The drawing under review shows one solid part. Ordinate dimensions are in mm from its lowest x, y, z. Coordinates: 2 decimals unless noted, no trailing zeros. Loops run counter-clockwise (first coordinate to the right, second up) from the corner with the lowest first, then second, coordinate; pieces in that order, holes last. Notation, with made-up numbers: (53, 15) -> (106, 15) arc R18 ccw to (106, 40) -> close; hole circle Ø4 at (22.5, 17). An arc over 180 degrees is marked (long way). Use a Markdown table: item, result.
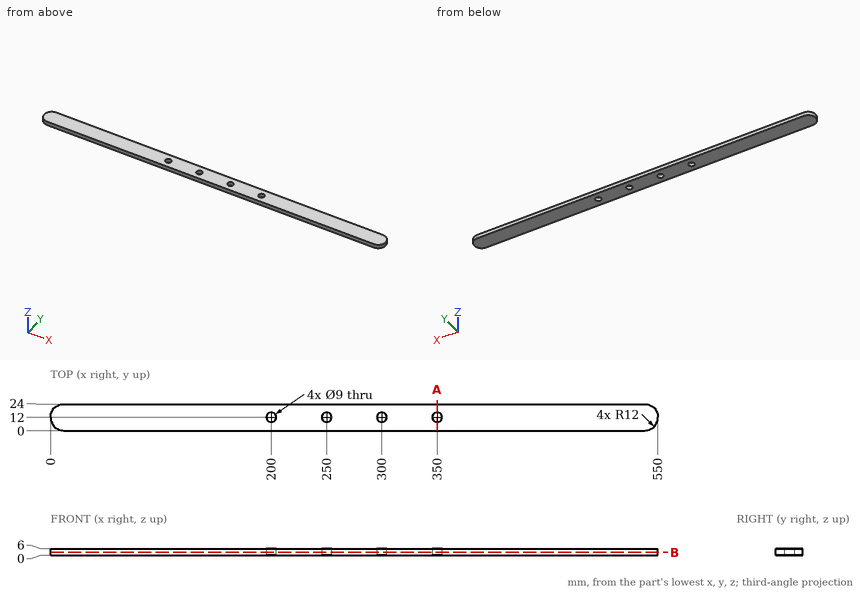
(1) Take a section at B-B on z = 2.45. State how many separate pieces and enclosed holes the cut face has, plus the area to 3 significant figures.
Found:
| item | result |
|---|---|
| separate pieces | 1 |
| enclosed holes | 4 |
| area | 12,800 mm^2 |
(2) For pin 1 Ø1.5 at (y, z) = (6.5, 3) entering from +X; pin 2 Ø1.5 at (y, z) = (16.5, 2.5) entering from -X, all flat-tipped, find the tip position at first contact; note any pin that passes through.
Found:
| item | result |
|---|---|
| pin 1 | stops at x = 549.02 |
| pin 2 | stops at x = 0.6 |
(3) Take a section at A-A on x = 350. Write out the cut boundary in (y, z), plus the area to 3 significant figures.
Found:
| item | result |
|---|---|
| outline | (0, 0) -> (7.5, 0) -> (7.5, 6) -> (0, 6) -> close; (16.5, 0) -> (24, 0) -> (24, 6) -> (16.5, 6) -> close |
| area | 90.0 mm^2 |
(4) For line 1 along X through (y, z) = (11.75, 1.35); line 2 along X through (y, z) = (12.75, 4.65); line 3 along Y through (x, z) = (200, 4.7), list the stretches that pass through material, from the lowest coordinate up.
Found:
| item | result |
|---|---|
| line 1 | x = 0 to 195.51, 204.49 to 245.51, 254.49 to 295.51, 304.49 to 345.51, 354.49 to 550 |
| line 2 | x = 0.02 to 195.56, 204.44 to 245.56, 254.44 to 295.56, 304.44 to 345.56, 354.44 to 549.98 |
| line 3 | y = 0 to 7.5, 16.5 to 24 |
